from build123d import *

# Parameters (mm, degrees)
SKETCH1_W               = 20
SKETCH1_H               = 20
SKETCH1_W_2             = 15
SKETCH1_H_2             = 6
SKETCH1_R               = 2
SKETCH1_W_3             = 6
SKETCH1_H_3             = 11.976495928
BOSS_EXTRUDE2_DEPTH     = 1.5
BOSS_EXTRUDE3_DEPTH     = 3.5
SKETCH3_W               = 10
SKETCH3_H               = 11.976495928
SKETCH3_W_2             = 15
SKETCH3_H_2             = 10
BOSS_EXTRUDE4_DEPTH     = 3.5
CUT_EXTRUDE1_DEPTH      = 38.878044984
CUT_EXTRUDE1_DEPTH_BACK = 38.878044984
SKETCH5_R               = 2
SKETCH6_W               = 1.5
SKETCH6_H               = 6
SKETCH6_W_2             = 6
SKETCH6_H_2             = 1.5
BOSS_EXTRUDE6_DEPTH     = 15
CHAMFER1_SIZE           = 3
CUT_EXTRUDE4_DEPTH      = 43.008883487
CUT_EXTRUDE4_DEPTH_BACK = 43.008883487
SKETCH7_R               = 2
CUT_EXTRUDE5_DEPTH      = 51.889549928
CUT_EXTRUDE5_DEPTH_BACK = 51.889549928
SKETCH8_R               = 2


with BuildPart() as part:
    # Sketch1 → Boss-Extrude2 (new body)
    # profile 1 of 3: a face of its own
    with BuildSketch(Plane(origin=(0, 0, 0), x_dir=(0, 0, -1), z_dir=(1, 0, 0))):
        with Locations((10, 21.976495928)):
            Rectangle(SKETCH1_W, SKETCH1_H)
    # profile 2 of 3: a face of its own
    with BuildSketch(Plane(origin=(0, 0, 0), x_dir=(0, 0, -1), z_dir=(1, 0, 0))):
        with Locations((-7.5, 21.976495928)):
            Rectangle(SKETCH1_W_2, SKETCH1_H_2)
        with Locations((-9.5, 21.976495928)):
            Circle(SKETCH1_R, mode=Mode.SUBTRACT)
    # profile 3 of 3: a face of its own
    with BuildSketch(Plane(origin=(0, 0, 0), x_dir=(0, 0, -1), z_dir=(1, 0, 0))):
        with Locations((10, 5.988247964)):
            Rectangle(SKETCH1_W_3, SKETCH1_H_3)
        with Locations((10, 5.5)):
            Circle(SKETCH1_R, mode=Mode.SUBTRACT)
    extrude(amount=BOSS_EXTRUDE2_DEPTH)

    # Sketch2 → Boss-Extrude3 (add)
    with BuildSketch(Plane.ZY):
        Polygon((-20, 31.976495928), (0, 31.976495928), (0, 24.976495928), (0, 11.976495928), (-20, 11.976495928), align=None)
    extrude(amount=BOSS_EXTRUDE3_DEPTH)

    # Sketch3 → Boss-Extrude4 (add)
    with BuildSketch(Plane.ZY):
        with Locations((-10, 5.988247964)):
            Rectangle(SKETCH3_W, SKETCH3_H)
        with Locations((7.5, 21.976495928)):
            Rectangle(SKETCH3_W_2, SKETCH3_H_2)
    extrude(amount=BOSS_EXTRUDE4_DEPTH)

    # Sketch5 → Cut-Extrude1 (cut, two sides: drawn at the far end of the back side and taken through both)
    with BuildSketch(Plane(origin=(0, 0, 0), x_dir=(0, 0, -1), z_dir=(1, 0, 0)).offset(-CUT_EXTRUDE1_DEPTH_BACK)):
        with Locations((-9.5, 21.976495928)):
            Circle(SKETCH5_R)
        with Locations((10, 5.5)):
            Circle(SKETCH5_R)
    extrude(amount=CUT_EXTRUDE1_DEPTH + CUT_EXTRUDE1_DEPTH_BACK, mode=Mode.SUBTRACT)

    # Sketch6 → Boss-Extrude6 (add)
    with BuildSketch(Plane.ZY.offset(3.5)):
        Polygon((-18.5, 26.976495928), (-18.5, 24.976495928), (-18.5, 18.976495928), (-18.5, 16.976495928), (-18, 16.976495928), (-15, 19.976495928), (-15, 23.976495928), (-18, 26.976495928), align=None)
        with Locations((-19.25, 21.976495928)):
            Rectangle(SKETCH6_W, SKETCH6_H)
        Polygon((-5, 29.976495928), (-5, 30.476495928), (-7, 30.476495928), (-13, 30.476495928), (-15, 30.476495928), (-15, 29.976495928), (-12, 26.976495928), (-8, 26.976495928), align=None)
        with Locations((-10, 31.226495928)):
            Rectangle(SKETCH6_W_2, SKETCH6_H_2)
    extrude(amount=BOSS_EXTRUDE6_DEPTH)

    # Chamfer1
    chamfer1_edges = [part.edges().sort_by_distance(p)[0] for p in [
        (-3.5, 5.988247964, -15),
        (-3.5, 5.988247964, -5),
        (-3.5, 16.976495928, 7.5),
        (-3.5, 26.976495928, 7.5),
    ]]
    chamfer(chamfer1_edges, length=CHAMFER1_SIZE - 0.0001)  # a hair under: the kernel refuses the full size

    # Sketch7 → Cut-Extrude4 (cut, two sides: drawn at the far end of the back side and taken through both)
    with BuildSketch(Plane(origin=(0, 31.976495928, 0), x_dir=(1, 0, 0), z_dir=(0, 1, 0)).offset(-CUT_EXTRUDE4_DEPTH_BACK)):
        with Locations(Location((-13, 10, 0), (0, 0, 270))):
            Circle(SKETCH7_R)
    extrude(amount=CUT_EXTRUDE4_DEPTH + CUT_EXTRUDE4_DEPTH_BACK, mode=Mode.SUBTRACT)

    # Sketch8 → Cut-Extrude5 (cut, two sides: drawn at the far end of the back side and taken through both)
    with BuildSketch(Plane(origin=(0, 0, -20), x_dir=(-1, 0, 0), z_dir=(0, 0, -1)).offset(-CUT_EXTRUDE5_DEPTH_BACK)):
        with Locations((13, 21.976495928)):
            Circle(SKETCH8_R)
    extrude(amount=CUT_EXTRUDE5_DEPTH + CUT_EXTRUDE5_DEPTH_BACK, mode=Mode.SUBTRACT)


solid = part.part
Read the model definition and answer for the solid it produces. Units are mm, in the model's axes. A direction names the side the tool comes from. Coordinates: 2 decimals unless noted, no trailing zeros. Order: outer loops, then holes, each group sorted by start corner. A loop starts at its lowest first (then second) coordinate and runs counter-clockwise, first axis right, second up. Notation, with made-up numbers: (12, -22) - (66, -22) arc R15 cw to (66, -1) - close; hole circle Ø5 at (87, -28). An arc over 180 degrees is marked (long way). Use one line per item in the form item = value.
(1) For a pull along X with two mould halves and no side action, classify faces 4 (the face through (-1.979, 18.455, 7.395)), 5 (the face through (-12.74, 23.96, -17.46)), 6 (the face through (0, 18, 7)), 7 (the face through (-11, 30.476, -6)) as pulls with the +X half, pulls with the -X half, needs draft (parallel to the pull), parting line crosses it, or undercut.
Computed values:
face_4 = pulls with the -X half
face_5 = undercut
face_6 = pulls with the +X half
face_7 = needs draft
(2) Which of the six approach directions +Z, -Z, +X, -X, +Y, -Y give full straight-line access (tool end or side, diameter ignored) to faces 1 (the face through (-10.895, 28.497, -13.521)), 2 (the face through (-16, 22, -15)), 3 (the face through (-11, 26, -18.5))?
Computed values:
face_1 = -Z, -X, -Y
face_2 = +Z, -X, -Y
face_3 = -Z, -X, +Y
(3) Straight lines are drawn through the part: L1, parallel to X at y = 28.2, z = -10; L2, parallel to Z at x = -13, y = 30.4; L3, parallel to X at y = 18.5, z = -1.5. For each, find the intervals that lie inside material, in ascending order.
Computed values:
L1 = -18.5 to -15, -11 to 1.5
L2 = -15 to -12, -8 to -5
L3 = -3.5 to 1.5
(4) Given pin 1 Ø8 at (x, y) = (-14, 12.5) entering from +Z; pin 2 Ø0.8 at (x, z) = (1, 7) entering from +Y; pin 3 Ø0.6 at (x, y) = (-10, 26) entering from -Z; pin 4 Ø1.6 at (x, y) = (-14, 31.5) entering from +Z, each flat-ended and moving along its own axis, determine where each tip first touches the part or whether it passes through.
Computed values:
pin_1 = through
pin_2 = 24.98
pin_3 = -18.5
pin_4 = -7
(5) Section C-C, the plane z = -10 is taken. Give the vertices of the cut face in (x, y), then the cut area to 3 significant figures.
Computed values:
outline = (-18.5, 26.98) - (-15, 26.98) - (-15, 31.98) - (-18.5, 31.98) - close; (-11, 26.98) - (-3.5, 26.98) - (-3.5, 7.5) - (1.5, 7.5) - (1.5, 31.98) - (-11, 31.98) - close; (-3.5, 0) - (1.5, 0) - (1.5, 3.5) - (-3.5, 3.5) - close
area = 195 mm²
(6) Section B-B, the plane x = -16.75 is taken. Give the vertices of the cut face in (y, z).
Computed values:
outline = (16.98, -18.5) - (18.98, -18.5) - (18.98, -20) - (24.98, -20) - (24.98, -18.5) - (26.98, -18.5) - (26.98, -18) - (23.98, -15) - (19.98, -15) - (16.98, -18) - close; (26.98, -12) - (29.98, -15) - (30.48, -15) - (30.48, -13) - (31.98, -13) - (31.98, -7) - (30.48, -7) - (30.48, -5) - (29.98, -5) - (26.98, -8) - close
